Job drawing, mm, ordinate dimensions from the low corner. One solid piece. A direction names the side the tool comes from. Give positions to 0.01 mm unless a question says otherwise; leave off trailing zeros. Order: outer loops, then holes, each group sorted by start corner. A loop starts at its lowest first (then second) coordinate and runs counter-clockwise, first axis right, second up.
Item 1: Wall check: L1, parallel to X at y = 3.5, z = 1.25; L2, parallel to Y at x = 2, z = 7.25; L3, parallel to Y at x = 2, z = 5.5. Give the ranges that are in metal, low to high.
Item 2: Band-saw the part on B-B on x = 1.8. Give the cut face in (y, z), plus the area to 3 significant figures.
Item 3: Which spindle directions (+Z, -Z, +X, -X, +Y, -Y) get a long thin tool onto all of the face, cutting with end or side? Do the marked faces 1 and 2. Say none if no direction does.
Item 4: Band-saw the part on C-C on z = 5. Give the cut face in (x, y).
Item 5: Two-plate mould, pull along Y, no slides. Class the marked faces 3, 4 and 5: released by +Y, released by -Y, zero draft, split by the parting line, or undercut.
Item 6: Band-saw the part on A-A on y = 3.59. Give the cut face in (x, z), plus the area to 3 significant figures.
Item 7: Band-saw the part on D-D on z = 3.25. Give the cut face in (x, y), plus the area to 3 significant figures.
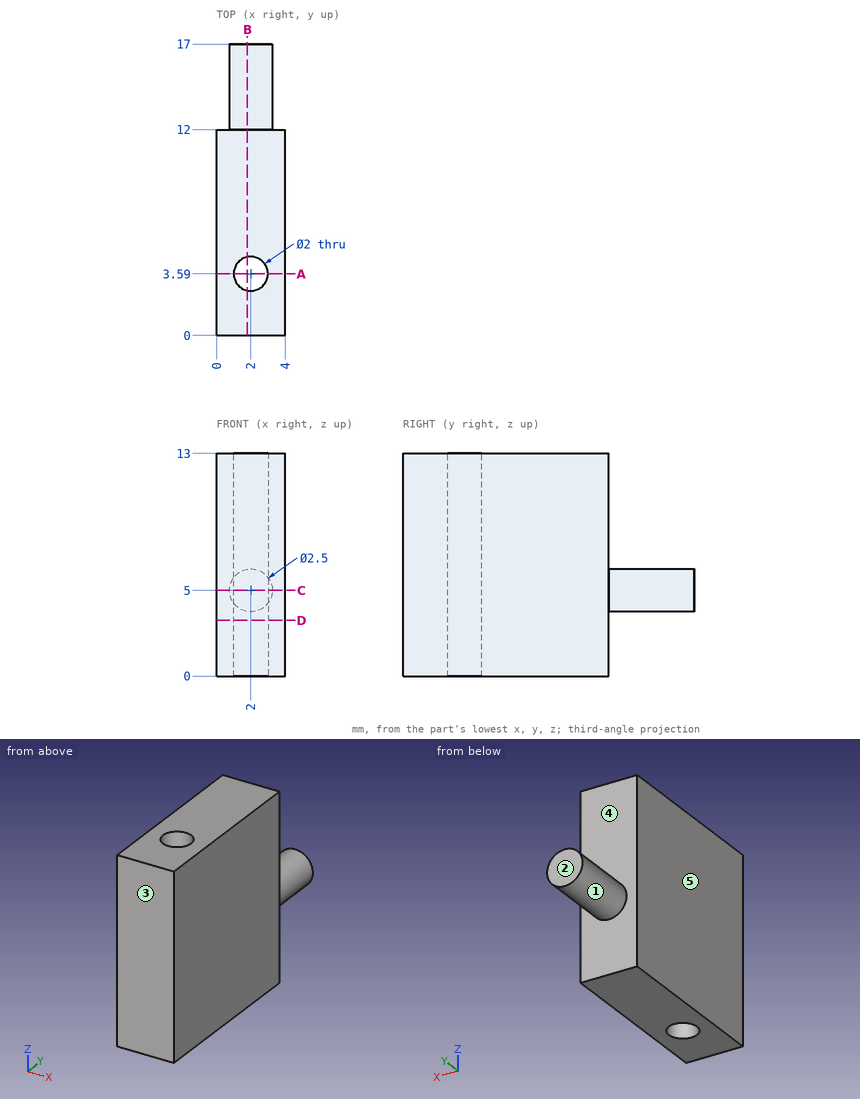
The answers:
1. L1: x = 0 to 1, 3 to 4
1. L2: y = 0 to 2.59, 4.59 to 12
1. L3: y = 0 to 2.59, 4.59 to 17
2. outline: (0, 0) - (2.61, 0) - (2.61, 13) - (0, 13) - close; (4.57, 0) - (12, 0) - (12, 3.77) - (17, 3.77) - (17, 6.23) - (12, 6.23) - (12, 13) - (4.57, 13) - close
2. area: 143 mm2
3. face 1: +Y
3. face 2: +Z, -Z, +X, -X, +Y
4. outline: (0, 0) - (4, 0) - (4, 12) - (3.25, 12) - (3.25, 17) - (0.75, 17) - (0.75, 12) - (0, 12) - close; hole circle Ø2 at (2, 3.59)
5. face 3: released by -Y
5. face 4: released by +Y
5. face 5: zero draft
6. outline: (0, 0) - (1, 0) - (1, 13) - (0, 13) - close; (3, 0) - (4, 0) - (4, 13) - (3, 13) - close
6. area: 26.0 mm2
7. outline: (0, 0) - (4, 0) - (4, 12) - (0, 12) - close; hole circle Ø2 at (2, 3.59)
7. area: 44.9 mm2
